Geometry: final body of the model. Coordinates: model frame, mm. A direction names the side the tool comes from. Give positions to 0.01 mm unless a question says otherwise; leave off trailing zeros. Write each loop counter-clockwise with the first axis right and the second up, starting at its lowest first coordinate (ties: lowest second). Pieces come first, ordered by that corner, then holes. Notation, with made-up numbers: (-16.5, 82.25) - (1.5, 82.25) arc R20 ccw to (1.5, 107.25) - close; hole circle Ø2 at (4.5, 18). An arc over 180 degrees is marked (long way). Return JSON: item names as keys, results as strings.
from build123d import *

# Parameters (mm, degrees)
SKETCH1_R            = 6
BOSS_EXTRUDE1_DEPTH  = 12
M6_CLEARANCE_HOLE1_D = 6.6


with BuildPart() as part:
    # Sketch1 → Boss-Extrude1 (new body)
    with BuildSketch(Plane(origin=(0, 0, 0), x_dir=(0, 0, -1), z_dir=(1, 0, 0))):
        Polygon((0, 0), (45, 0), (45, 20), (29, 20), (29, 5), (0, 5), align=None)
        with Locations((37, 12)):
            Circle(SKETCH1_R, mode=Mode.SUBTRACT)
    extrude(amount=BOSS_EXTRUDE1_DEPTH)

    # M6 Clearance Hole1 (through all)
    with Locations(Plane(origin=(0, 5, 0), x_dir=(-1, 0, 0), z_dir=(0, 1, 0))):
        with Locations((-6, -20)):
            Hole(M6_CLEARANCE_HOLE1_D / 2)


solid = part.part
Q1. Pin query (flat end, axial travel): P1, Ø3, axis at x = 5.5, z = -24, coming from the +Y side. Return the tip coordinate at first contact, or that it passes through.
Answer key:
{"P1": "stops at y = 5"}
Q2. Mould query, pull axis Z, two halves, no side actions, for faces 3 (the cylindrical face through (5.92, 8.35, -32.24)), 4 (the flat face through (6, 10, -45)), 5 (the flat face through (6, 3, 0)), 6 (the flat face through (6, 5, -15)). Classes: pulls with the +Z half, pulls with the -Z half, needs draft (parallel to the pull), parting line crosses it, or undercut.
Answer key:
{"face 3": "undercut", "face 4": "pulls with the -Z half", "face 5": "pulls with the +Z half", "face 6": "needs draft"}
Q3. Section query C-C, the plane x = 6. Return the cut outline in (y, z), plus the area to 3 significant figures.
Answer key:
{"outline": "(0, -45) - (20, -45) - (20, -29) - (5, -29) - (5, -23.3) - (0, -23.3) - close; (0, -16.7) - (5, -16.7) - (5, 0) - (0, 0) - close; hole circle Ø12 at (12, -37)", "area": "319 mm^2"}
Q4. Section query A-A, the plane z = -20. Return the cut outline in (x, y), plus the area to 3 significant figures.
Answer key:
{"outline": "(0, 0) - (2.7, 0) - (2.7, 5) - (0, 5) - close; (9.3, 0) - (12, 0) - (12, 5) - (9.3, 5) - close", "area": "27.0 mm^2"}
Q5. Section query D-D, the plane y = 3. Return the cut outline in (x, z).
Answer key:
{"outline": "(0, -45) - (12, -45) - (12, 0) - (0, 0) - close; hole circle Ø6.6 at (6, -20)"}
Q6. Set-up query: faces 1 (the cylindrical face through (3.381, 2.465, -22.008)), 2 (the flat face through (6, 13, -29)). Return all of +Z, -Z, +X, -X, +Y, -Y with unobstructed straight access to the full face (end or side cutting, diameter ignored); none if empty.
Answer key:
{"face 1": "+Y, -Y", "face 2": "+Z, +X, -X, +Y"}
Q7. Material intervals for probe 1 along Z at (x, y) = (7, 12.25); probe 2 along Z at (x, y) = (6, 3.5); probe 3 along Y at (x, z) = (3.5, -37), sorted ascending. Write a range as [from, to].
Answer key:
{"probe 1": "z = [-45, -42.99], [-31.01, -29]", "probe 2": "z = [-45, -23.3], [-16.7, 0]", "probe 3": "y = [0, 6], [18, 20]"}
Q8. Section query B-B, the plane y = 12. Return the cut outline in (x, z), plus the area to 3 significant figures.
Answer key:
{"outline": "(0, -45) - (12, -45) - (12, -43) - (0, -43) - close; (0, -31) - (12, -31) - (12, -29) - (0, -29) - close", "area": "48.0 mm^2"}
